For this review, take the finished solid that the model builds, in its own axes (mm). A direction names the side the tool comes from. Give positions to 0.01 mm unless a question says otherwise; leave off trailing zeros. Write each loop counter-clockwise with the first axis right and the second up, starting at its lowest first coordinate (ties: lowest second). Pieces come first, ordered by that corner, then holes. Notation, with made-up numbers: (15, -9.75) -> (25, -9.75) arc R28 ccw to (25, 19.25) -> close; hole circle Ø3 at (-20.75, -18). An arc over 180 degrees is marked (long way). Write item = value, one per line.
```python
from build123d import *

# Parameters (mm, degrees)
SKETCH1_R           = 15
BOSS_EXTRUDE2_DEPTH = 40
SKETCH1_4_R         = 15
SKETCH1_4_R_2       = 13
BOSS_EXTRUDE3_DEPTH = 3
CUT_EXTRUDE1_DEPTH  = 291.688837075


with BuildPart() as part:
    # Sketch1 → Boss-Extrude2 (new body)
    with BuildSketch(Plane(origin=(0, 0, 0), x_dir=(1, 0, 0), z_dir=(0, 1, 0))):
        with BuildLine():
            Line((-13.228756555, 95), (-175, 95))
            Line((-175, 95), (-175, 70))
            Line((-175, 70), (-95, 70))
            Line((-95, 70), (-95, -70))
            Line((-95, -70), (-175, -70))
            Line((-175, -70), (-175, -95))
            Line((-175, -95), (-13.228756555, -95))
            ThreePointArc((-13.228756555, -95), (0, -100), (13.228756555, -95))
            Line((13.228756555, -95), (175, -95))
            Line((175, -95), (175, 95))
            Line((175, 95), (13.228756555, 95))
            ThreePointArc((13.228756555, 95), (0, 100), (-13.228756555, 95))
        make_face()
        with Locations(Location((0, -80, 0), (0, 0, 270))):
            Circle(SKETCH1_R, mode=Mode.SUBTRACT)
        with Locations(Location((0, 80, 0), (0, 0, 270))):
            Circle(SKETCH1_R, mode=Mode.SUBTRACT)
    extrude(amount=-BOSS_EXTRUDE2_DEPTH)

    # Sketch1_4 → Boss-Extrude3 (add)
    # profile 1 of 2: a face of its own
    with BuildSketch(Plane(origin=(0, 0, 0), x_dir=(1, 0, 0), z_dir=(0, 1, 0))):
        with Locations(Location((0, 80, 0), (0, 0, 270))):
            Circle(SKETCH1_4_R)
        with Locations(Location((0, 80, 0), (0, 0, 270))):
            Circle(SKETCH1_4_R_2, mode=Mode.SUBTRACT)
    # profile 2 of 2: a face of its own
    with BuildSketch(Plane(origin=(0, 0, 0), x_dir=(1, 0, 0), z_dir=(0, 1, 0))):
        with Locations(Location((0, -80, 0), (0, 0, 270))):
            Circle(SKETCH1_4_R)
        with Locations(Location((0, -80, 0), (0, 0, 270))):
            Circle(SKETCH1_4_R_2, mode=Mode.SUBTRACT)
    extrude(amount=-BOSS_EXTRUDE3_DEPTH)

    # Sketch3 → Cut-Extrude1 (cut, through all)
    with BuildSketch(Plane.ZY.offset(95)):
        Polygon((-58, -40), (-56.5, -10), (-53.5, -10), (-52, -40), align=None)
        Polygon((-48, -40), (-46.5, -10), (-43.5, -10), (-42, -40), align=None)
        Polygon((-38, -40), (-36.5, -10), (-33.5, -10), (-32, -40), align=None)
        Polygon((-28, -40), (-26.5, -10), (-23.5, -10), (-22, -40), align=None)
        Polygon((-18, -40), (-16.5, -10), (-13.5, -10), (-12, -40), align=None)
        Polygon((-8, -40), (-6.5, -10), (-3.5, -10), (-2, -40), align=None)
        Polygon((2, -40), (3.5, -10), (6.5, -10), (8, -40), align=None)
        Polygon((12, -40), (13.5, -10), (16.5, -10), (18, -40), align=None)
        Polygon((22, -40), (23.5, -10), (26.5, -10), (28, -40), align=None)
        Polygon((32, -40), (33.5, -10), (36.5, -10), (38, -40), align=None)
        Polygon((42, -40), (43.5, -10), (46.5, -10), (48, -40), align=None)
        Polygon((52, -40), (53.5, -10), (56.5, -10), (58, -40), align=None)
    extrude(amount=-CUT_EXTRUDE1_DEPTH, mode=Mode.SUBTRACT)


solid = part.part
```
(1) Take a section at B-B (x = -146). Write out the cut boundary in (y, z), plus the area to 3 significant figures.
Answers below:
outline = (-40, -95) -> (0, -95) -> (0, -70) -> (-40, -70) -> close; (-40, 70) -> (0, 70) -> (0, 95) -> (-40, 95) -> close
area = 2,000 mm^2
(2) For pin 1 (6 mm diameter, centred on x = -66.5, y = -19.5, fed in from +Z); pin 2 (6 mm diameter, centred on x = -67.5, z = 20, fed in from +Y); pin 3 (3 mm diameter, centred on y = -10, z = 5, fed in from -X); pin 4 (1.5 mm diameter, centred on x = 77.5, z = -34.5, fed in from -Y), all flat-tipped, find the tip position at first contact; note any pin that passes through.
Answers below:
pin_1 = 95
pin_2 = 0
pin_3 = -95
pin_4 = -10
(3) Take a section at A-A (z = 80). Write out the cut boundary in (x, y), plus the area to 3 significant figures.
Answers below:
outline = (-175, -40) -> (-15, -40) -> (-15, -3) -> (-13, -3) -> (-13, 0) -> (-175, 0) -> close; (13, -3) -> (15, -3) -> (15, -40) -> (175, -40) -> (175, 0) -> (13, 0) -> close
area = 12,800 mm^2
(4) Take a section at C-C (y = -27). Count the separate pieces of the cut face and the enclosed holes in it, plus the area to 3 significant figures.
Answers below:
separate_pieces = 13
enclosed_holes = 2
area = 38,800 mm^2
(5) The part is to be moulded in two halves that separate along Z. For faces 1 (the face through (38.11, -24.79, 57.24)), 2 (the face through (-175, -20, -83)), 3 (the face through (0, -20, -100)), say which applies: released by +Z, released by -Z, zero draft, split by the parting line, or undercut.
Answers below:
face_1 = undercut
face_2 = zero draft
face_3 = released by -Z
(6) To check wall thickness, follow probe 1 along X at (y, z) = (-1, -80); probe 2 along X at (y, z) = (-24.5, -73.5); probe 3 along X at (y, z) = (-38, -21). State the ranges of each line that lie inside material, in increasing order.
Answers below:
probe_1 = -175 to -13, 13 to 175
probe_2 = -175 to -13.52, 13.52 to 175
probe_3 = -95 to 175
(7) Tool access review of faces 4 (the face through (38.11, -25.21, 2.74)), 5 (the face through (12.65, -21.24, -71.94)), 6 (the face through (0.572, -1.479, 67.013)), 7 (the face through (-136, -20, -70)), 8 (the face through (41, 0, -1)): name each direction out of +Z, -Z, +X, -X, +Y, -Y from which nothing blocks a thin tool from reaching the whole face with its end or side.
Answers below:
face_4 = +X, -X, -Y
face_5 = -Y
face_6 = +Y, -Y
face_7 = -X, +Y, -Y
face_8 = +Z, -Z, +X, -X, +Y
